The model under review builds one solid part; all positions refer to its coordinate system, in mm. A direction names the side the tool comes from. Coordinates: 2 decimals unless noted, no trailing zeros. Write each loop counter-clockwise with the first axis right and the second up, starting at its lowest first coordinate (ties: lowest second). Pieces come first, ordered by that corner, then holes. Notation, with made-up numbers: M 9.5,52 L 16.5,52 A16 ccw 16.5,80 Z; hole C 75.5,41.25 d5. An arc over 180 degrees is marked long. Answer as a JSON object with one key per item and string values.
```python
from build123d import *

# Parameters (mm, degrees)
F0_R            = 2
F1_DEPTH        = 10
F2_W            = 6
F2_H            = 20
F3_DEPTH        = 20
F4_R            = 2.15
F5_DEPTH        = 25
F6_R            = 6
F8_D            = 4
F8_DEPTH        = 7
F8_CSINK_D      = 7
F8_CSINK_ANGLE  = 90
F10_D           = 4
F10_DEPTH       = 12
F10_CSINK_D     = 7
F10_CSINK_ANGLE = 90


with BuildPart() as f1:
    # F0 (on Top) → F1 (new body)
    with BuildSketch(Plane.XY):
        with Locations((12.5, 0)):
            Circle(F0_R)
        Polygon((17.5, 0), (17.5, 10), (-17.5, 10), (-17.5, -10), (17.5, -10), align=None)
        with Locations((12.5, 0)):
            Circle(F0_R, mode=Mode.SUBTRACT)
    extrude(amount=-F1_DEPTH)

    # F2 (on face) → F3 (join)
    with BuildSketch(Plane.XY):
        with Locations((2.5, 0)):
            Rectangle(F2_W, F2_H)
    extrude(amount=F3_DEPTH)

    # F4 (on face) → F5 (cut)
    with BuildSketch(Plane.YZ.offset(5.5)):
        with Locations((0, 12)):
            Circle(F4_R)
    extrude(amount=-F5_DEPTH, mode=Mode.SUBTRACT)

    # F6
    f6_edges = [f1.edges().sort_by_distance(p)[0] for p in [
        (2.5, -10, 20),
        (2.5, 10, 20),
        (17.5, 10, -5),
        (17.5, -10, -5),
    ]]
    fillet(f6_edges, radius=F6_R)

    # F8
    with Locations(Plane.YZ.offset(5.5)):
        with Locations((0, 12)):
            CounterSinkHole(F8_D / 2, F8_CSINK_D / 2, depth=F8_DEPTH, counter_sink_angle=F8_CSINK_ANGLE)

    # F10
    with Locations(Plane.XY):
        with Locations((12.5, 0)):
            CounterSinkHole(F10_D / 2, F10_CSINK_D / 2, depth=F10_DEPTH, counter_sink_angle=F10_CSINK_ANGLE)


solid = f1.part
```
(1) Add section A-A on z = 12. Give the boundary of the cut face in (x, y), and give its area (3 significant figures).
Results list:
{"outline": "M -0.5,-10 L 5.5,-10 L 5.5,-3.5 L 4.15,-2.15 L -0.5,-2.15 Z; M -0.5,2.15 L 4.15,2.15 L 5.5,3.5 L 5.5,10 L -0.5,10 Z", "area": "92.4 mm²"}
(2) For pin 1 Ø1.5 at (x, y) = (-12.5, 3) entering from +Z; pin 2 Ø5 at (y, z) = (0, 12) entering from +X; pin 3 Ø3.5 at (x, y) = (11.5, -1) entering from +Z, all flat-tipped, find the tip position at first contact; note any pin that passes through.
Results list:
{"pin 1": "z = 0", "pin 2": "x = 4.5", "pin 3": "z = -0.34"}
(3) Draft analysis for pull direction Z (two halves, no side actions). For faces 4 (the face through (5.5, 0, 8)), 5 (the face through (1.858, -1.706, 10.692)), 6 (the face through (-9, 0, 0)), 7 (the face through (0, 0, -10)), state which applies: released by +Z, released by -Z, zero draft, split by the parting line, or undercut.
Results list:
{"face 4": "zero draft", "face 5": "undercut", "face 6": "released by +Z", "face 7": "released by -Z"}
(4) Add section C-C on x = 12.5. Give the boundary of the cut face in (y, z).
Results list:
{"outline": "M -9.92,-10 L -2,-10 L -2,-1.5 L -3.5,0 L -9.92,0 Z; M 2,-10 L 9.92,-10 L 9.92,0 L 3.5,0 L 2,-1.5 Z"}
(5) For faces 1 (the face through (-0.5, 0, 8)), 2 (the face through (-17.5, 0, -5)), 3 (the face through (8.7, 0.1, 0)), list the 3-axis set-ups (+Z, -Z, +X, -X, +Y, -Y) from which the entire face can be reached by the end or side of a thin tool; tool diameter is ignored.
Results list:
{"face 1": "+Z, -X, +Y, -Y", "face 2": "+Z, -Z, -X, +Y, -Y", "face 3": "+Z, +X, +Y, -Y"}
(6) Wall thickness on line 1 along Y through (x, z) = (1, 12); line 2 along X through (y, z) = (0, -4.75); line 3 along X through (y, z) = (-6, 12): over which ranges is each line inside the solid? List them lowest first. Write a range as from..to.
Results list:
{"line 1": "-10..-2.15, 2.15..10", "line 2": "-17.5..10.5, 14.5..17.5", "line 3": "-0.5..5.5"}
(7) Add section B-B on y = 0. Give the boundary of the cut face in (x, z).
Results list:
{"outline": "M -17.5,-10 L 10.5,-10 L 10.5,-1.5 L 9,0 L 5.5,0 L 5.5,8.5 L 4.15,9.85 L -0.5,9.85 L -0.5,0 L -17.5,0 Z; M -0.5,14.15 L 4.15,14.15 L 5.5,15.5 L 5.5,20 L -0.5,20 Z; M 14.5,-10 L 17.5,-10 L 17.5,0 L 16,0 L 14.5,-1.5 Z"}
(8) Add section D-D on z = -3.5. Give the boundary of the cut face in (x, y), and give its area (3 significant figures).
Results list:
{"outline": "M -17.5,-10 L 11.5,-10 A6 ccw 17.5,-4 L 17.5,4 A6 ccw 11.5,10 L -17.5,10 Z; hole C 12.5,0 d4", "area": "672 mm²"}
